Design review of the part built by this model. Coordinates are the model's own, in mm. A direction names the side the tool comes from. Round coordinates to 2 decimals unless told otherwise and drop trailing zeros. Order: outer loops, then holes, each group sorted by start corner. A loop starts at its lowest first (then second) coordinate and runs counter-clockwise, first axis right, second up.
from build123d import *

# Parameters (mm, degrees)
SKETCH1_W            = 45.2
SKETCH1_H            = 20.6
BOSS_EXTRUDE1_DEPTH  = 1.1
SKETCH2_R            = 7.95
BOSS_EXTRUDE2_DEPTH  = 12.1
BOSS_EXTRUDE3_DEPTH  = 2.6
SKETCH5_W            = 10.591964238
SKETCH5_H            = 2.906134497
SKETCH5_W_2          = 9.8
SKETCH5_H_2          = 2.3
CUT_EXTRUDE2_DEPTH   = 0.1
SKETCH6_W            = 0.5
SKETCH6_H            = 0.5
SKETCH8_W            = 0.5
SKETCH8_H            = 0.5
BOSS_EXTRUDE4_DEPTH  = 0.5
BOSS_EXTRUDE4_TAPER  = 10
LPATTERN1_COUNT      = 4
LPATTERN1_PITCH      = 2.5
SKETCH9_R            = 6.55
CUT_EXTRUDE3_DEPTH   = 10
SKETCH10_R           = 5.35
BOSS_EXTRUDE5_DEPTH  = 1
SKETCH11_R           = 3.55
BOSS_EXTRUDE6_DEPTH  = 1
BOSS_EXTRUDE10_DEPTH = 0.7
BOSS_EXTRUDE11_DEPTH = 2.8
SKETCH18_R           = 1
CUT_EXTRUDE4_DEPTH   = 7.45
SKETCH19_R           = 0.5
BOSS_EXTRUDE12_DEPTH = 2.6
CUT_EXTRUDE5_DEPTH   = 0.1
FILLET1_R            = 0.5
SKETCH33_R           = 6.55
BOSS_EXTRUDE21_DEPTH = 0.1
FILLET4_R            = 0.2


with BuildPart() as part:
    # Sketch1 → Boss-Extrude1 (new body)
    with BuildSketch(Plane(origin=(0, 0, 0), x_dir=(1, 0, 0), z_dir=(0, 1, 0))):
        Rectangle(SKETCH1_W, SKETCH1_H)
    extrude(amount=BOSS_EXTRUDE1_DEPTH)

    # Sketch2 → Boss-Extrude2 (add)
    with BuildSketch(Plane(origin=(0, 1.1, 0), x_dir=(1, 0, 0), z_dir=(0, 1, 0))):
        with Locations((12.8, 0)):
            Circle(SKETCH2_R)
        with Locations((-12.8, 0)):
            Circle(SKETCH2_R)
    extrude(amount=BOSS_EXTRUDE2_DEPTH)

    # Sketch3 → Boss-Extrude3 (add)
    with BuildSketch(Plane.XZ):
        Polygon((-4.58, 10.3), (-5.08, 9.8), (-5.08, 8.3), (-4.58, 7.8), (-3.04, 7.8), (-2.54, 8.3), (-2.04, 7.8), (-0.5, 7.8), (0, 8.3), (0.5, 7.8), (2.04, 7.8), (2.54, 8.3), (3.04, 7.8), (4.58, 7.8), (5.08, 8.3), (5.08, 9.8), (4.58, 10.3), (3.04, 10.3), (2.54, 9.8), (2.04, 10.3), (0.5, 10.3), (0, 9.8), (-0.5, 10.3), (-2.04, 10.3), (-2.54, 9.8), (-3.04, 10.3), align=None)
    extrude(amount=BOSS_EXTRUDE3_DEPTH)

    # Sketch5 → Cut-Extrude2 (cut)
    with BuildSketch(Plane.XZ):
        with Locations((0, 9.071641639)):
            Rectangle(SKETCH5_W, SKETCH5_H)
        with Locations((0, 9.05)):
            Rectangle(SKETCH5_W_2, SKETCH5_H_2, mode=Mode.SUBTRACT)
    extrude(amount=CUT_EXTRUDE2_DEPTH, mode=Mode.SUBTRACT)

    # Sweep1: sweep along a path in Sketch7
    with BuildLine(Plane(origin=(-3.81, 0, 0), x_dir=(0, 0, -1), z_dir=(1, 0, 0))) as sweep1_path:
        Line((-9.05, -2.6), (-9.05, -4.6))
        ThreePointArc((-9.05, -4.6), (-9.196446609, -4.953553391), (-9.55, -5.1))
        Line((-9.55, -5.1), (-14.95, -5.1))
    # Sketch6 → Sweep1 (sweep)
    with BuildSketch(Plane.XZ.offset(2.6)):
        with Locations((-3.81, 9.05)):
            Rectangle(SKETCH6_W, SKETCH6_H)
    sweep1 = sweep(path=sweep1_path.line)

    # Sketch8 → Boss-Extrude4 (add)
    with BuildSketch(Plane.XY.offset(14.95)):
        with Locations((-3.81, -5.1)):
            Rectangle(SKETCH8_W, SKETCH8_H)
    boss_extrude4 = extrude(amount=BOSS_EXTRUDE4_DEPTH, taper=BOSS_EXTRUDE4_TAPER)

    # LPattern1: Sweep1, Boss-Extrude4 ×4
    with Locations(*[(i * LPATTERN1_PITCH, 0, 0) for i in range(1, LPATTERN1_COUNT)]):
        add(sweep1)
        add(boss_extrude4)

    # Sketch9 → Cut-Extrude3 (cut)
    with BuildSketch(Plane(origin=(0, 13.2, 0), x_dir=(1, 0, 0), z_dir=(0, 1, 0))):
        with Locations((12.8, 0)):
            Circle(SKETCH9_R)
    cut_extrude3 = extrude(amount=-CUT_EXTRUDE3_DEPTH, mode=Mode.SUBTRACT)

    # Sketch10 → Boss-Extrude5 (add)
    with BuildSketch(Plane(origin=(0, 3.2, 0), x_dir=(1, 0, 0), z_dir=(0, 1, 0))):
        with Locations((12.8, 0)):
            Circle(SKETCH10_R)
    boss_extrude5 = extrude(amount=BOSS_EXTRUDE5_DEPTH)

    # Sketch11 → Boss-Extrude6 (add)
    with BuildSketch(Plane(origin=(0, 4.2, 0), x_dir=(1, 0, 0), z_dir=(0, 1, 0))):
        with Locations((12.8, 0)):
            Circle(SKETCH11_R)
    boss_extrude6 = extrude(amount=BOSS_EXTRUDE6_DEPTH)

    # Mirror1: Cut-Extrude3, Boss-Extrude5, Boss-Extrude6 across plane
    add(cut_extrude3.mirror(Plane(origin=(0, 0, 0), x_dir=(0, 0, 1), z_dir=(1, 0, 0))), mode=Mode.SUBTRACT)
    add(boss_extrude5.mirror(Plane(origin=(0, 0, 0), x_dir=(0, 0, 1), z_dir=(1, 0, 0))))
    add(boss_extrude6.mirror(Plane(origin=(0, 0, 0), x_dir=(0, 0, 1), z_dir=(1, 0, 0))))

    # Sketch16 → Boss-Extrude10 (add)
    with BuildSketch(Plane(origin=(0, 1.1, 0), x_dir=(1, 0, 0), z_dir=(0, 1, 0))):
        with BuildLine():
            Line((-2.85, 10.3), (2.85, 10.3))
            ThreePointArc((2.85, 10.3), (5.05, 8.1), (2.85, 5.9))
            Line((2.85, 5.9), (-2.85, 5.9))
            ThreePointArc((-2.85, 5.9), (-5.05, 8.1), (-2.85, 10.3))
        make_face()
    extrude(amount=BOSS_EXTRUDE10_DEPTH)

    # Sketch17 → Boss-Extrude11 (add)
    with BuildSketch(Plane(origin=(0, 1.8, 0), x_dir=(1, 0, 0), z_dir=(0, 1, 0))):
        with BuildLine():
            Line((-2.85, 9.85), (2.85, 9.85))
            ThreePointArc((2.85, 9.85), (4.6, 8.1), (2.85, 6.35))
            Line((2.85, 6.35), (-2.85, 6.35))
            ThreePointArc((-2.85, 6.35), (-4.6, 8.1), (-2.85, 9.85))
        make_face()
    extrude(amount=BOSS_EXTRUDE11_DEPTH)

    # Sketch18 → Cut-Extrude4 (cut, through all)
    with BuildSketch(Plane(origin=(0, 1.1, 0), x_dir=(1, 0, 0), z_dir=(0, 1, 0))):
        with Locations((-21.2, -8.9)):
            Circle(SKETCH18_R)
        with Locations((21.2, 8.9)):
            Circle(SKETCH18_R)
    extrude(amount=-CUT_EXTRUDE4_DEPTH, mode=Mode.SUBTRACT)

    # Sketch19 → Boss-Extrude12 (add)
    with BuildSketch(Plane.XZ):
        with Locations((-12.8, 4.65)):
            Circle(SKETCH19_R)
        with Locations((-12.8, -4.65)):
            Circle(SKETCH19_R)
        with Locations((12.8, -4.65)):
            Circle(SKETCH19_R)
        with Locations((12.8, 4.65)):
            Circle(SKETCH19_R)
    extrude(amount=BOSS_EXTRUDE12_DEPTH)

    # Sketch20 → Cut-Extrude5 (cut)
    with BuildSketch(Plane(origin=(0, 1.1, 0), x_dir=(1, 0, 0), z_dir=(0, 1, 0))):
        with BuildLine():
            Line((-2.85, 5.9), (2.85, 5.9))
            ThreePointArc((2.85, 5.9), (5.05, 8.1), (2.85, 10.3))
            Line((2.85, 10.3), (-2.85, 10.3))
            ThreePointArc((-2.85, 10.3), (-5.05, 8.1), (-2.85, 5.9))
        make_face()
        with BuildLine():
            Line((-2.85, 6), (2.85, 6))
            ThreePointArc((2.85, 6), (4.95, 8.1), (2.85, 10.2))
            Line((2.85, 10.2), (-2.85, 10.2))
            ThreePointArc((-2.85, 10.2), (-4.95, 8.1), (-2.85, 6))
        make_face(mode=Mode.SUBTRACT)
    extrude(amount=CUT_EXTRUDE5_DEPTH, mode=Mode.SUBTRACT)

    # Fillet1
    fillet1_edges = [part.edges().sort_by_distance(p)[0] for p in [
        (4.85, 13.2, 0),
        (-20.75, 13.2, 0),
    ]]
    fillet(fillet1_edges, radius=FILLET1_R)

    # Sketch33 → Boss-Extrude21 (add)
    with BuildSketch(Plane(origin=(0, 12.7, 0), x_dir=(1, 0, 0), z_dir=(0, 1, 0))):
        with Locations((12.8, 0)):
            Circle(SKETCH33_R)
    boss_extrude21 = extrude(amount=BOSS_EXTRUDE21_DEPTH)

    # Mirror2: Boss-Extrude21 across plane
    add(boss_extrude21.mirror(Plane(origin=(0, 0, 0), x_dir=(0, 0, 1), z_dir=(1, 0, 0))))

    # Fillet4
    fillet4_edges = [part.edges().sort_by_distance(p)[0] for p in [
        (-4.6, 1.8, -8.1),
        (0, 1.8, -6.35),
        (4.6, 1.8, -8.1),
        (0, 1.8, -9.85),
        (-4.6, 4.6, -8.1),
        (0, 4.6, -6.35),
        (4.6, 4.6, -8.1),
        (0, 4.6, -9.85),
    ]]
    fillet(fillet4_edges, radius=FILLET4_R)


solid = part.part
1) For faces 1 (the face through (7, 3.2, 0)), 2 (the face through (0, 4.6, -8)), 3 (the face through (-5.217, 6.819, -2.388)), 4 (the face through (4, -1, 10.3)), 5 (the face through (-4.06, -5, 11)), list the 3-axis set-ups (+Z, -Z, +X, -X, +Y, -Y) from which the entire face can be reached by the end or side of a thin tool; tool diameter is ignored.
Results:
face 1: none
face 2: +Z, -Z, +Y
face 3: +Y
face 4: +Z, +X, -X, +Y
face 5: +Z, -Z, -X, -Y
2) Take a section at A-A on x = -21.2. Give the boundary of the cut face in (y, z).
Results:
outline: (0, -10.3) - (1.1, -10.3) - (1.1, 7.9) - (0, 7.9) - close; (0, 9.9) - (1.1, 9.9) - (1.1, 10.3) - (0, 10.3) - close
3) Take a section at B-B on z = 13. Give the boundary of the cut face in (x, y).
Results:
outline: (-4.06, -5.35) - (-3.56, -5.35) - (-3.56, -4.85) - (-4.06, -4.85) - close; (-1.56, -5.35) - (-1.06, -5.35) - (-1.06, -4.85) - (-1.56, -4.85) - close; (0.94, -5.35) - (1.44, -5.35) - (1.44, -4.85) - (0.94, -4.85) - close; (3.44, -5.35) - (3.94, -5.35) - (3.94, -4.85) - (3.44, -4.85) - close
4) Take a section at C-C on y = 6.5. Give the boundary of the cut face in (x, z).
Results:
outline: circle Ø15.9 at (-12.8, 0); circle Ø15.9 at (12.8, 0); hole circle Ø13.1 at (-12.8, 0); hole circle Ø13.1 at (12.8, 0)
5) To check wall thickness, follow line 1 along X through (y, z) = (0.7, -8.9); line 2 along X through (y, z) = (0.8, 8.9); line 3 along Z through (x, y) = (-21.2, 0.3). State the ranges of each line that lie inside material, in increasing order.
Results:
line 1: x = -22.6 to 20.2, 22.2 to 22.6
line 2: x = -22.6 to -22.2, -20.2 to 22.6
line 3: z = -10.3 to 7.9, 9.9 to 10.3
6) The part is to be moulded in two halves that separate along Z. For faces 6 (the face through (-7, 3.2, 0)), 7 (the face through (22.6, 0.5, 0.1)), 8 (the face through (-1, -1, 10.3)), say which applies: released by +Z, released by -Z, zero draft, split by the parting line, or undercut.
Results:
face 6: undercut
face 7: zero draft
face 8: released by +Z
7) Clearance check with flat-ended pins moving along their axes: P1, Ø4, axis at x = 3.5, z = -3.5, coming from the -Y side; P2, Ø1.5, axis at y = 5.5, z = -2, coming from the +X side; P3, Ø3, axis at y = -4, z = 11.5, coming from the -X side; P4, Ø5, axis at y = -3, z = 1.5, coming from the +X side. State where each tip first meets the part, or that it passes through.
Results:
P1: stops at y = 0
P2: stops at x = 20.65
P3: stops at x = -4.06
P4: passes through
